Geometry: see drawing. Coordinates: mm, zero at the bounding-box minimum. A direction names the side the tool comes from. Round coordinates to 2 decimals unless told otherwise and drop trailing zeros. Order: outer loops, then holes, each group sorted by start corner. A loop starts at its lowest first (then second) coordinate and runs counter-clockwise, first axis right, second up. Notation, with made-up numbers: M 58.5,48 L 92.5,48 A20 cw 92.5,74 Z; hole C 51.25,43.25 d1. An arc over 180 degrees is marked long. Answer in a Markdown table with one row per item. Add a question column.
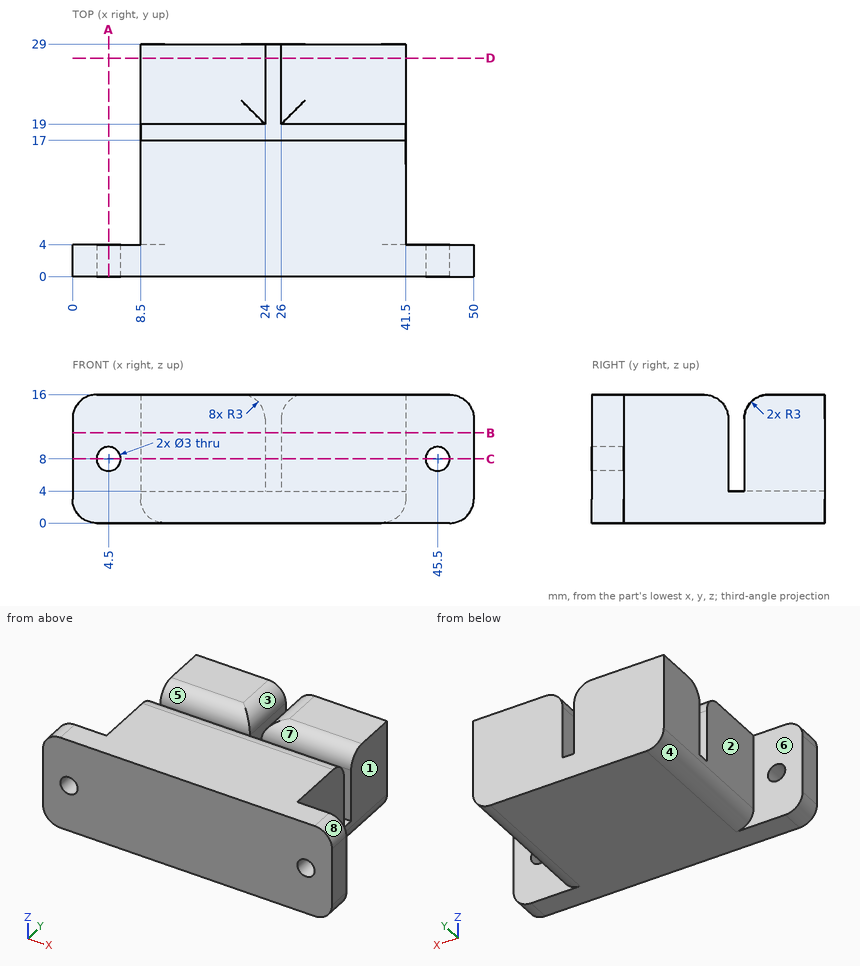
(1) Cut plane D-D (y = 27.25). Return loops of the section in (x, z), and give its area (3 significant figures).
(2) Line query: line 1 (Y direction, x = 16.5, z = 13); line 2 (Z direction, x = 4.5, y = 2.95); line 3 (X direction, y = 26, z = 13.25). Output: solid intervals per line, ascending. Write a range as from..to.
(3) Pin query (flat end, axial travel): pin 1 (5 mm diameter, centred on x = 45.5, z = 8, fed in from +Y); pin 2 (2.5 mm diameter, centred on y = 26, z = 7, fed in from +X); pin 3 (1 mm diameter, centred on y = 14, z = 12, fed in from -X). Return the tip coordinate at first contact, or that it passes through.
(4) Draft query along Y for the marked faces 5, 6, 7 and 8. Return one class per face: +Y half, -Y half, draft (parallel to the pull), parting line (faces both ways), or undercut.
(5) Cut plane C-C (z = 8). Return loops of the section in (x, y).
(6) Cut plane A-A (x = 4.5). Return loops of the section in (y, z).
(7) Access query for the marked faces 1, 2, 3 and 4. Directions: +Z, -Z, +X, -X, +Y, -Y. A direction counts if a zero-diameter tool reaches every point of the face in a straight line with its end or side. Return the directions, or none.
(8) Cut plane B-B (z = 11.25). Return loops of the section in (x, y), and give its area (3 significant figures).
Answer list:
| question | item | result |
|---|---|---|
| 1 | outline | M 8.5,3 A3 ccw 11.5,0 L 38.5,0 A3 ccw 41.5,3 L 41.5,16 L 29,16 A3 ccw 26,13 L 26,4 L 24,4 L 24,13 A3 ccw 21,16 L 8.5,16 Z |
| 1 | area | 496 mm² |
| 2 | line 1 | 0..17, 19..29 |
| 2 | line 2 | 0..6.5, 9.5..16 |
| 2 | line 3 | 8.5..23.99, 26.01..41.5 |
| 3 | pin 1 | y = 4 |
| 3 | pin 2 | x = 41.5 |
| 3 | pin 3 | x = 8.5 |
| 4 | face 5 | undercut |
| 4 | face 6 | +Y half |
| 4 | face 7 | undercut |
| 4 | face 8 | draft |
| 5 | outline | M 0,0 L 3,0 L 3,4 L 0,4 Z; M 6,0 L 44,0 L 44,4 L 41.5,4 L 41.5,17 L 8.5,17 L 8.5,4 L 6,4 Z; M 8.5,19 L 24,19 L 24,29 L 8.5,29 Z; M 26,19 L 41.5,19 L 41.5,29 L 26,29 Z; M 47,0 L 50,0 L 50,4 L 47,4 Z |
| 6 | outline | M 0,0 L 4,0 L 4,6.5 L 0,6.5 Z; M 0,9.5 L 4,9.5 L 4,16 L 0,16 Z |
| 7 | face 1 | +Z, -Z, +X, +Y |
| 7 | face 2 | +Z, -Z, -X, +Y |
| 7 | face 3 | +Z, +Y |
| 7 | face 4 | -Z, -X, +Y |
| 8 | outline | M 0,0 L 50,0 L 50,4 L 41.5,4 L 41.5,17 L 8.5,17 L 8.5,4 L 0,4 Z; M 8.5,19 L 24,19 L 24,29 L 8.5,29 Z; M 26,19 L 41.5,19 L 41.5,29 L 26,29 Z |
| 8 | area | 939 mm² |
